Model file for the job. Use its own axes, mm. Coordinates: 2 decimals unless noted, no trailing zeros. Write each loop counter-clockwise with the first axis right and the second up, starting at its lowest first coordinate (ties: lowest second). Pieces come first, ordered by that corner, then holes. Notation, with made-up numbers: (-12, 12) - (30, 12) arc R26 cw to (30, 32) - close; hole circle Ø9 at (1, 61.25). An arc over 180 degrees is marked (long way). Put each result on its own line as item: value. Start each with the question number.
1. Saw through at B-B, the plane z = -190. Write the cut outline in (x, y), plus the area to 3 significant figures.
2. Saw through at A-A, the plane y = 8.75. Write the cut outline in (x, z).
3. Saw through at C-C, the plane x = 150. Write the cut outline in (y, z).
4. Drill centre lines: L1, parallel to Z at x = 82, y = 6; L2, parallel to X at y = 3.75, z = -190; L3, parallel to Z at x = 64, y = 6.75. Where is each one in solid material? Low to high. Write a range as from..to.
5. Drop flat-ended pins along their axis: P1, Ø1.9, axis at x = 82, z = -215, coming from the -Y side; P2, Ø6, axis at y = 5, z = 7, coming from the -X side; P3, Ø3.5, axis at y = 5, z = 3, coming from the +X side. Give the stop position or say it passes through.
6. Saw through at D-D, the plane x = 22.5. Write the cut outline in (y, z).
```python
from build123d import *

# Parameters (mm, degrees)
SALIENTE_EXTRUIR1_DEPTH = 12
CROQUIS2_R              = 1.55
CROQUIS2_R_2            = 3.9
CORTAR_EXTRUIR1_DEPTH   = 12
REDONDEO1_R             = 70


with BuildPart() as part:
    # Croquis1 → Saliente-Extruir1 (new body)
    with BuildSketch(Plane(origin=(0, 0, 0), x_dir=(1, 0, 0), z_dir=(0, 1, 0))):
        Polygon((0, 0), (20, 0), (20, -12), (48, -12), (48, 0), (68, 0), (68, -12), (96, -12), (96, 0), (116, 0), (116, -12), (144, -12), (144, 0), (164, 0), (164, 230), (0, 230), align=None)
    extrude(amount=SALIENTE_EXTRUIR1_DEPTH)

    # Croquis2 → Cortar-Extruir1 (cut)
    with BuildSketch(Plane(origin=(0, 12, 0), x_dir=(1, 0, 0), z_dir=(0, 1, 0))):
        with Locations(Location((82, 215, 0), (0, 0, 270))):
            Circle(CROQUIS2_R)
        with Locations(Location((57, 155, 0), (0, 0, 270))):
            Circle(CROQUIS2_R)
        with Locations(Location((107, 155, 0), (0, 0, 270))):
            Circle(CROQUIS2_R)
        with Locations(Location((62, 190, 0), (0, 0, 270))):
            Circle(CROQUIS2_R_2)
        with Locations(Location((102, 190, 0), (0, 0, 270))):
            Circle(CROQUIS2_R_2)
    extrude(amount=-CORTAR_EXTRUIR1_DEPTH, mode=Mode.SUBTRACT)

    # Redondeo1
    redondeo1_edges = [part.edges().sort_by_distance(p)[0] for p in [
        (164, 6, -230),
        (0, 6, -230),
    ]]
    fillet(redondeo1_edges, radius=REDONDEO1_R)


solid = part.part
```
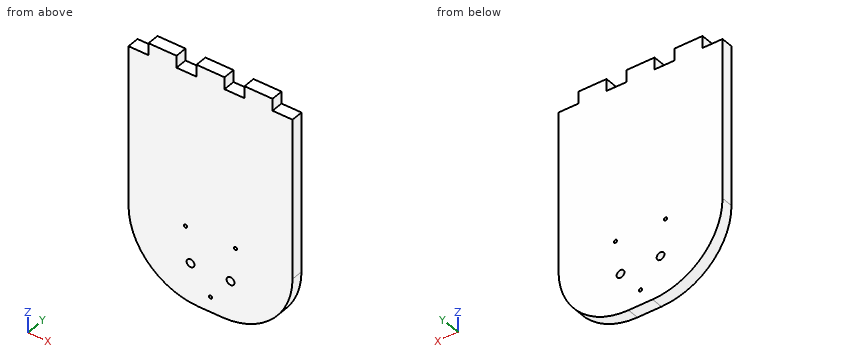
Final values:
1. outline: (6.75, 0) - (58.1, 0) - (58.1, 12) - (6.75, 12) - close; (65.9, 0) - (98.1, 0) - (98.1, 12) - (65.9, 12) - close; (105.9, 0) - (157.25, 0) - (157.25, 12) - (105.9, 12) - close
1. area: 1,620 mm²
2. outline: (0, -160) arc R70 ccw to (70, -230) - (94, -230) arc R70 ccw to (164, -160) - (164, 0) - (144, 0) - (144, 12) - (116, 12) - (116, 0) - (96, 0) - (96, 12) - (68, 12) - (68, 0) - (48, 0) - (48, 12) - (20, 12) - (20, 0) - (0, 0) - close; hole circle Ø3.1 at (57, -155); hole circle Ø7.8 at (62, -190); hole circle Ø3.1 at (82, -215); hole circle Ø7.8 at (102, -190); hole circle Ø3.1 at (107, -155)
3. outline: (0, -202) - (12, -202) - (12, 0) - (0, 0) - close
4. L1: z = -230..-216.55, -213.45..12
4. L2: x = 6.75..58.1, 65.9..98.1, 105.9..157.25
4. L3: z = -229.74..-193.35, -186.65..0
5. P1: passes through
5. P2: stops at x = 20
5. P3: stops at x = 144
6. outline: (0, -211.42) - (12, -211.42) - (12, 12) - (0, 12) - close
